Part model, mm, in its own coordinate system. Face numbers are marked on the shaded views. A direction names the side the tool comes from. Round coordinates to 2 decimals unless told otherwise and drop trailing zeros. Order: outer loops, then holes, each group sorted by start corner. A loop starts at its lowest first (then second) coordinate and runs counter-clockwise, first axis right, second up. Notation, with made-up numbers: M -39,30.5 L 17,30.5 A9 cw 17,36.5 Z; hole C 48,35.5 d8. An arc over 180 degrees is marked long. Write each question's results on one line, items separated by ' | '. Start each with the question number.
1. Which spindle directions (+Z, -Z, +X, -X, +Y, -Y) get a long thin tool onto all of the face, cutting with end or side? Do the marked faces 5 and 6. Say none if no direction does.
2. Drop flat-ended pins along their axis: pin 1 Ø1 at (x, z) = (31, -1) entering from -Y; pin 2 Ø3 at (x, z) = (-25, -5) entering from +Y; pin 3 Ø0.9 at (x, y) = (0, 3) entering from +Z; pin 4 Ø6 at (x, z) = (29, 5) entering from -Y. Give the stop position or say it passes through.
3. Two-plate mould, pull along X, no slides. Class the marked faces 1, 2, 3 and 4: +X half, -X half, draft (parallel to the pull), parting line (faces both ways), or undercut.
4. Band-saw the part on B-B, the plane y = 1.25. Give the number of separate pieces and of enclosed holes in the cut face, then the cut area to 3 significant figures.
5. Band-saw the part on A-A, the plane x = -28.5. List the corners of the cut face in (y, z), then the cut area to 3 significant figures.
6. Probe L1, parallel to X at y = 3, z = -5; L2, parallel to X at y = 6.5, z = 2; L3, parallel to X at y = 7, z = -2.5. List the from-to ranges inside material, lowest first. Write a range as [from, to].
7. Band-saw the part on C-C, the plane z = -6. List the corners of the cut face in (x, y) (3 decimals), then the cut area to 3 significant figures.
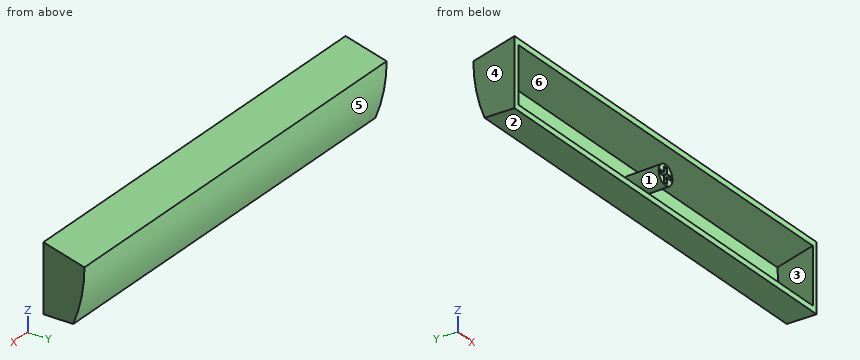
Autodesk Inventor part; units mm, degrees
ref_plane "PoleBase Plane" through (57, 9.4826, 4.9062) normal (0, 0.9995, -0.0304) x (-1, 0, 0)
ref_plane "YZ Plane" through (0, 0, 0) normal (1, 0, 0) x (0, 1, 0)
ref_plane "XZ Plane" through (0, 0, 0) normal (0, 1, 0) x (-1, 0, 0)
sketch "Spacebar base" plane through (0, 0, 0) normal (0, 1, 0) x (-1, 0, 0)
  line L0 (58.5, 9) -> (-58.5, 9)
  line L1 (-58.5, 9) -> (-58.5, -9)
  line L2 (-58.5, -9) -> (58.5, -9)
  line L3 (58.5, -9) -> (58.5, 9)
  line L4 (58.5, 9) -> (-58.5, -9) construction
  line L5 (-58.5, 9) -> (58.5, -9) construction
  point P0 (0, 0)
  dimension "d0" = 117
  dimension "d1" = 18
extrude "Spacebar Bulk" add sketch "Spacebar base" along normal blind 11
sketch "Curve Profile" plane through (58.5, 0, 9) normal (1, 0, 0) x (0, 0, -1)
  line L0 (0, 0) -> (18, 0)
  line L1 (0, 0) -> (2.9474, 11)
  line L2 (0, 11) -> (18, 11)
  line L3 (18, 0) -> (18, 11)
  arc A0 (18, 8) -> (2.9474, 11) centre (2.9474, -28.2633) ccw
  line L4 (0, 0) -> (0, 11)
  line L5 (18, 8) -> (18, 0)
  line L6 (18, 0) -> (0, 0)
  point P0 (9, 0)
  dimension "d4" = 15
  dimension "d9" = 8
extrude "Curve Cutaway" cut sketch "Curve Profile" against normal up to surface (117 mm away) contours L1 A0 L3 L0 keep common part
shell "Inner Shell" thickness 1.5 removed faces 1 at (19.5, 0, 3)
ref_plane "PoleBase Plane" through (57, 9.4826, 4.9062) normal (0, 0.9995, -0.0304) x (-1, 0, 0)
sketch "Center Circle" plane through (57, 9.4826, 4.9062) normal (0, 0.9995, -0.0304) x (-1, 0, 0)
  circle A0 centre (57, -5.1918) radius 2.65
  dimension "d11" = 5.3
extrude "Pole Extrusion" add sketch "Center Circle" against normal up to surface surface through (0, 0, 0) normal (0, 1, 0)
sketch "Sketch4" plane through (0, 0, 0) normal (0, -1, 0) x (1, 0, 0)
  line L0 (-2.075, 0.55) -> (2.075, 0.55)
  line L1 (2.075, 0.55) -> (2.075, -0.55)
  line L2 (2.075, -0.55) -> (-2.075, -0.55)
  line L3 (-2.075, -0.55) -> (-2.075, 0.55)
  line L4 (-2.075, 0.55) -> (2.075, -0.55) construction
  line L5 (2.075, 0.55) -> (-2.075, -0.55) construction
  line L6 (0.55, 2.075) -> (-0.55, 2.075)
  line L7 (-0.55, 2.075) -> (-0.55, -2.075)
  line L8 (-0.55, -2.075) -> (0.55, -2.075)
  line L9 (0.55, -2.075) -> (0.55, 2.075)
  line L10 (0.55, 2.075) -> (-0.55, -2.075) construction
  line L11 (-0.55, 2.075) -> (0.55, -2.075) construction
  point P0 (0, 0)
  dimension "d14" = 4.15
  dimension "d15" = 1.1
  dimension "d16" = 1.1
  dimension "d17" = 4.15
extrude "Extrusion4" cut sketch "Sketch4" against normal blind 5
equation "\"d0\" = b_space"
equation "\"d1\" = k_width"
equation "\"d10\" = k_wthick"
equation "\"d11\" = k_poledia"
equation "\"d14\" = k_cmxl"
equation "\"d15\" = k_cmxw"
equation "\"d16\" = k_cmxw"
equation "\"d17\" = k_cmxl"
equation "\"k_width\" = 18"
equation "\"k_height\" = 16.5"
equation "\"k_height_t\" = 16"
equation "\"k_taper1\" = 1.5"
equation "\"k_taper2\" = 0.5"
equation "\"k_staper\" = 1"
equation "\"k_sradius\" = 4"
equation "\"k_ltaper\" = 1.5"
equation "\"k_lradius\" = 6"
equation "\"k_radius\" = 6"
equation "\"k_wthick\" = 1.5"
equation "\"k_ribthick\" = 1.5"
equation "\"k_ribheight\" = 5"
equation "\"k_poleoff\" = 2.25"
equation "\"k_poledia\" = 5.3"
equation "\"k_cmxw\" = 1.1"
equation "\"k_cmxl\" = 4.15"
equation "\"s_bwidth\" = 14.4"
equation "\"s_poleh\" = 3.6"
equation "\"s_polebw\" = 5.4"
equation "\"s_polebl\" = 7.45"
equation "\"b_pad\" = 1"
equation "\"b_tab\" = 27"
equation "\"b_caps\" = 31.5"
equation "\"b_lshift\" = 40.5"
equation "\"b_rshift\" = 49.5"
equation "\"b_ctrl\" = 22.5"
equation "\"b_space\" = 117"
equation "\"b_width\" = 285"
equation "\"b_height\" = 77"
equation "\"k_taper_wide\" = 1.5"
equation "\"k_height_low\" = 15"
equation "\"k_taper_thin\" = 0.0001"
equation "\"k_shortening\" = 4.5"
equation "\"k_cmxd\" = 4"
equation "\"k_taper_side\" = 0.5"
properties part number "spacebar-keycap_mockup_cherrymx"
Solution:
1) face 5: -Z, +X, -X, +Y | face 6: -Y
2) pin 1: y = 8.74 | pin 2: y = 9.82 | pin 3: z = 8.32 | pin 4: y = 0
3) face 1: undercut | face 2: draft | face 3: undercut | face 4: -X half
4) separate pieces: 2 | enclosed holes: 2 | area: 415 mm^2
5) outline: M 0,-9 L 8,-9 A39.26 ccw 11,6.05 L 0,9 L 0,7.45 L 9.48,4.91 A37.76 cw 6.98,-7.5 L 0,-7.5 Z | area: 48.3 mm^2
6) L1: [-58.5, -57], [57, 58.5] | L2: [-58.5, -57], [-1.48, 1.48], [57, 58.5] | L3: [-58.5, -57], [-1.34, 1.34], [57, 58.5]
7) outline: M -58.5,0 L -57,0 L -57,7.525 L 57,7.525 L 57,0 L 58.5,0 L 58.5,9.104 L -58.5,9.104 Z | area: 207 mm^2
